Read the model definition and answer for the solid it produces. Units are mm, in the model's axes. Coordinates: 2 decimals unless noted, no trailing zeros. Write each loop counter-clockwise with the first axis right and the second up, starting at its lowest first coordinate (ties: lowest second). Pieces come first, ordered by that corner, then holes.
(1) Given pin 1 (1.5 mm diameter, centred on y = -4, z = 99, fed in from -X); pin 2 (2 mm diameter, centred on y = 4, z = 109.5, fed in from -X), each flat-ended and moving along its own axis, determine where each tip first touches the part or whether it passes through.
(2) Straight lines are drawn through the part: line 1 along Y through (x, z) = (0, 57.5) (3 decimals); line 2 along Y through (x, z) = (1.75, 10.5); line 3 along X through (y, z) = (0.5, 145). For each, find the intervals that lie inside material, in ascending order.
(3) The part is cut by section B-B, the plane z = 29. Determine the outline of the cut face in (x, y) (3 decimals), and give its area (3 significant figures).
(4) The part is cut by section A-A, the plane x = 0. Determine the outline of the cut face in (y, z) (3 decimals), and give its area (3 significant figures).
(5) The part is cut by section C-C, the plane y = 4.75. Determine the outline of the cut face in (x, z) (3 decimals).
(6) Determine the mould class of faces 1 (the flat face through (2, 3, 0)), 2 (the cylindrical face through (-0.69, -3.1, 85.32)), 3 (the flat face through (-5.525, 3.131, 82.96)) for opening direction X: pulls with the +X half, pulls with the -X half, needs draft (parallel to the pull), parting line crosses it, or undercut.
Autodesk Inventor part; units mm, degrees
ref_plane "YZ Plane" through (0, 0, 0) normal (1, 0, 0) x (0, 1, 0)
ref_plane "XZ Plane" through (0, 0, 0) normal (0, 1, 0) x (-1, 0, 0)
ref_plane "XY Plane" through (0, 0, 0) normal (0, 0, 1) x (1, 0, 0)
sketch "Sketch1" plane through (0, 0, 0) normal (0, 0, 1) x (1, 0, 0)
  line L0 (7.3323, 0) -> (3.6662, -6.35)
  line L1 (3.6662, -6.35) -> (-3.6662, -6.35)
  line L2 (-3.6662, -6.35) -> (-7.3323, 0)
  line L3 (-7.3323, 0) -> (-3.6662, 6.35)
  line L4 (-3.6662, 6.35) -> (3.6662, 6.35)
  line L5 (3.6662, 6.35) -> (7.3323, 0)
  point P0 (0, 0)
  point P1 (0, 0)
  dimension "d0" = 12.7
extrude "Extrusion1" add sketch "Sketch1" along normal blind 168.275
sketch "Sketch2" plane through (0, 0, 168.275) normal (0, 0, 1) x (1, 0, 0)
  circle A0 centre (0, 0) radius 3.175
  dimension "d3" = 6.35
extrude "Extrusion2" cut sketch "Sketch2" against normal blind 203.2
properties part number "wheel hex shaft"
Computed:
1. pin 1: stops at x = -5.46
1. pin 2: stops at x = -5.6
2. line 1: y = -6.35 to -3.175, 3.175 to 6.35
2. line 2: y = -6.35 to -2.65, 2.65 to 6.35
2. line 3: x = -7.04 to -3.14, 3.14 to 7.04
3. outline: (-7.332, 0) - (-3.666, -6.35) - (3.666, -6.35) - (7.332, 0) - (3.666, 6.35) - (-3.666, 6.35) - close; hole circle Ø6.35 at (0, 0)
3. area: 108 mm2
4. outline: (-6.35, 0) - (-3.175, 0) - (-3.175, 168.275) - (-6.35, 168.275) - close; (3.175, 0) - (6.35, 0) - (6.35, 168.275) - (3.175, 168.275) - close
4. area: 1,070 mm2
5. outline: (-4.59, 0) - (4.59, 0) - (4.59, 168.275) - (-4.59, 168.275) - close
6. face 1: needs draft
6. face 2: undercut
6. face 3: pulls with the -X half
